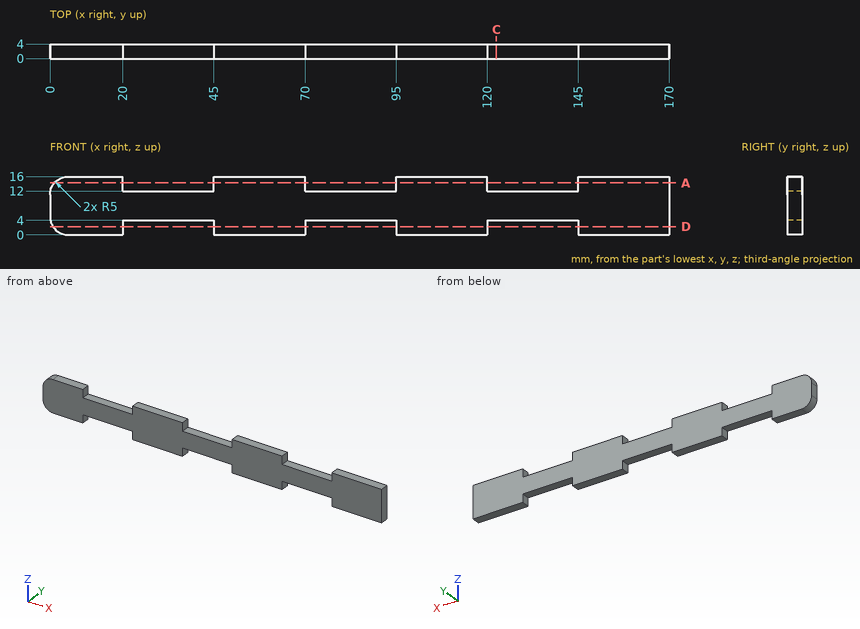
For this review, use the dimensioned drawing (mm, ordinates from the lowest corner) and the shaded views. Round coordinates to 2 decimals unless told otherwise and drop trailing zeros. Write each loop counter-clockwise with the first axis right and the second up, starting at its lowest first coordinate (ties: lowest second). Pieces come first, ordered by that corner, then holes. Notation, with made-up numbers: M -22.75,-6.5 L -2.75,-6.5 A35 cw -2.75,28.5 Z; hole C -30.75,-20 d6. An arc over 180 degrees is marked long. Use CSV: the item, a comma, the result in double quotes. Start each with the question number.
(1) We need section A-A, the plane z = 14.25. State the section outline as (x, y) points, then the cut area to 3 significant figures.
(2) We need section C-C, the plane x = 122.5. State the section outline as (y, z) points.
(3) For line 1 along X through (y, z) = (1.5, 3.5); line 2 along X through (y, z) = (0.45, 13.5); line 3 along Z through (x, y) = (23.5, 2.5), list the stretches that pass through material, from the lowest coordinate up.
(4) Clearance check with flat-ended pins moving along their axes: P1, Ø1.2, axis at x = 88, y = 2.5, coming from the -Z side; P2, Ø2, axis at y = 1.5, z = 14.5, coming from the -X side; P3, Ø1.2, axis at y = 1.5, z = 15, coming from the -X side. State where each tip first meets the part, or that it passes through.
(5) We need section D-D, the plane z = 2.25. State the section outline as (x, y) points, then the cut area to 3 significant figures.
Findings:
1,outline,"M 1.2,0 L 20,0 L 20,4 L 1.2,4 Z; M 45,0 L 70,0 L 70,4 L 45,4 Z; M 95,0 L 120,0 L 120,4 L 95,4 Z; M 145,0 L 170,0 L 170,4 L 145,4 Z"
1,area,"375 mm^2"
2,outline,"M 0,4 L 4,4 L 4,12 L 0,12 Z"
3,line 1,"0.23 to 20, 45 to 70, 95 to 120, 145 to 170"
3,line 2,"0.67 to 20, 45 to 70, 95 to 120, 145 to 170"
3,line 3,"4 to 12"
4,P1,"z = 4"
4,P2,"x = 0.67"
4,P3,"x = 1.33"
5,outline,"M 0.82,0 L 20,0 L 20,4 L 0.82,4 Z; M 45,0 L 70,0 L 70,4 L 45,4 Z; M 95,0 L 120,0 L 120,4 L 95,4 Z; M 145,0 L 170,0 L 170,4 L 145,4 Z"
5,area,"377 mm^2"
